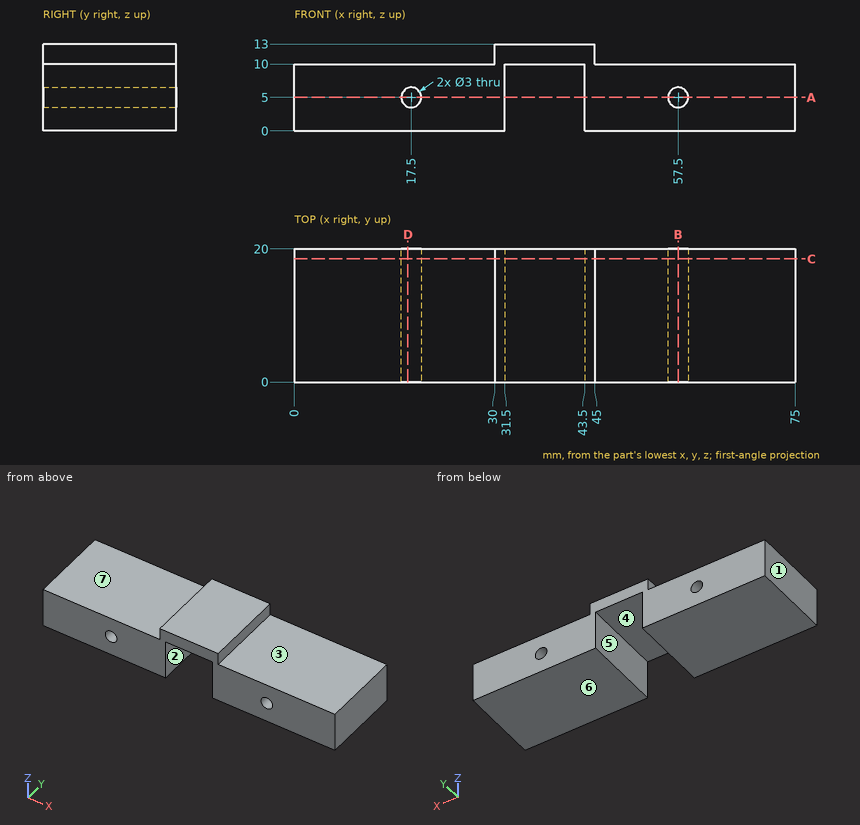
Verification items for this drawing (mm, ordinates from the low corner). A direction names the side the tool comes from. Give positions to 0.01 mm unless a question says otherwise; leave off trailing zeros. Loops run counter-clockwise (first coordinate to the right, second up) from the corner with the lowest first, then second, coordinate; pieces in that order, holes last. Notation, with made-up numbers: M 83.25,14.5 L 92.25,14.5 A6 ccw 92.25,20.5 Z; hole C 16.25,-3.5 d3. An arc over 180 degrees is marked long. Return JSON: item names as keys, results as strings. Group by question number.
1. Tool access check on the marked faces 5, 6 and 7. Record the directions out of +Z, -Z, +X, -X, +Y, -Y that give a thin tool (end or side, any length) a straight path to the whole face; none if there is none.
2. Cross-section at B-B on x = 57.5. Record the boundary of the cut face in (y, z), plus the area to 3 significant figures.
3. Cross-section at A-A on z = 5. Record the boundary of the cut face in (x, y), plus the area to 3 significant figures.
4. Cross-section at C-C on y = 18.5. Record the boundary of the cut face in (x, z).
5. Cross-section at D-D on x = 17. Record the boundary of the cut face in (y, z).
6. Mould release check, pull along X, two halves, no side actions. Record for the marked faces 1, 2, 3 and 4: released by +X, released by -X, zero draft, split by the parting line, or undercut.
7. Thickness scan on L1, parallel to X at y = 15.5, z = 1.5; L2, parallel to Z at x = 57.5, y = 6.25; L3, parallel to X at y = 1.5, z = 4. Record the ranges inside material, lowest first.
8. Go/stop test with flat-tipped pins: pin 1 (10 mm diameter, centred on x = 60.5, y = 9, fed in from +Z); pin 2 (2.5 mm diameter, centred on x = 57.5, z = 5, fed in from +Y); pin 3 (1.5 mm diameter, centred on y = 10, z = 11, fed in from +X); pin 4 (6 mm diameter, centred on x = 37.5, y = 13.5, fed in from -Z). Record where each tip stops, or that it passes through.
Return value:
{
 "1": {"face 5": "-Z, +Y, -Y", "face 6": "-Z, +X, -X, +Y, -Y", "face 7": "+Z, -X, +Y, -Y"},
 "2": {"outline": "M 0,0 L 20,0 L 20,3.5 L 0,3.5 Z; M 0,6.5 L 20,6.5 L 20,10 L 0,10 Z", "area": "140 mm^2"},
 "3": {"outline": "M 0,0 L 16,0 L 16,20 L 0,20 Z; M 19,0 L 31.5,0 L 31.5,20 L 19,20 Z; M 43.5,0 L 56,0 L 56,20 L 43.5,20 Z; M 59,0 L 75,0 L 75,20 L 59,20 Z", "area": "1,140 mm^2"},
 "4": {"outline": "M 0,0 L 31.5,0 L 31.5,10 L 43.5,10 L 43.5,0 L 75,0 L 75,10 L 45,10 L 45,13 L 30,13 L 30,10 L 0,10 Z; hole C 17.5,5 d3; hole C 57.5,5 d3"},
 "5": {"outline": "M 0,0 L 20,0 L 20,3.59 L 0,3.59 Z; M 0,6.41 L 20,6.41 L 20,10 L 0,10 Z"},
 "6": {"face 1": "released by -X", "face 2": "undercut", "face 3": "zero draft", "face 4": "undercut"},
 "7": {"L1": "0 to 31.5, 43.5 to 75", "L2": "0 to 3.5, 6.5 to 10", "L3": "0 to 16.38, 18.62 to 31.5, 43.5 to 56.38, 58.62 to 75"},
 "8": {"pin 1": "z = 10", "pin 2": "through", "pin 3": "x = 45", "pin 4": "z = 10"}
}
